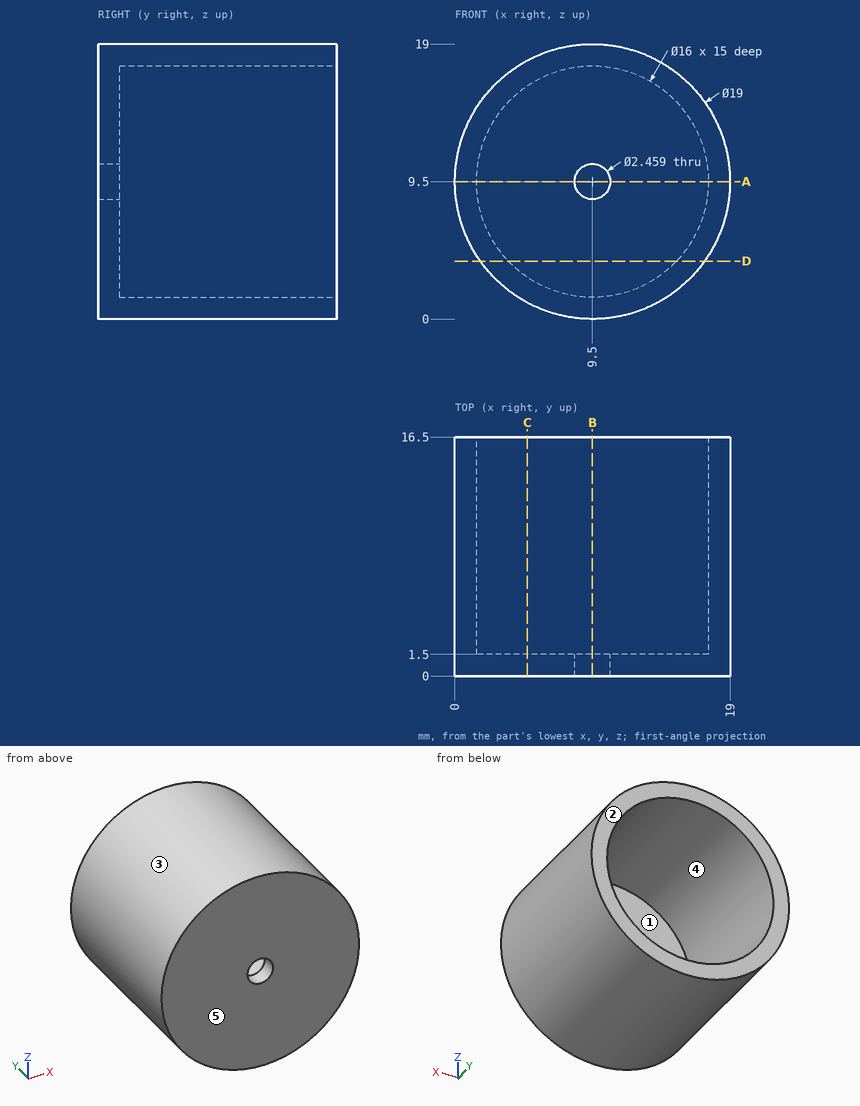
Study the drawing (mm; zero at the part's minimum x, y, z) and answer. A direction names the side the tool comes from. Give positions to 0.01 mm unless a question says otherwise; leave off trailing zeros. Write each loop counter-clockwise with the first axis right and the second up, starting at its lowest first coordinate (ties: lowest second). Pieces come first, ordered by that corner, then holes. Notation, with made-up numbers: M 45.25,88 L 52.25,88 A29 ccw 52.25,115 Z; hole C -5,27 d2. An arc over 180 degrees is marked long. Put each result on its own line as item: value. Start each with the question number.
1. The part is cut by section D-D, the plane z = 4. Give the vertices of the cut face in (x, y), and give its area (3 significant figures).
2. The part is cut by section C-C, the plane x = 5. Give the vertices of the cut face in (y, z), and give its area (3 significant figures).
3. Consider line 1 along Z through (x, y) = (9.5, 0.6); line 2 along Y through (x, z) = (11.5, 12); line 3 along Z through (x, y) = (9.5, 11.25). Determine where each line is inside the solid, lowest interval first.
4. Each of these flat-tipped pins is pushed along its axis until it touches: pin 1 Ø1.5 at (x, y) = (7, 2) entering from -Z; pin 2 Ø1 at (x, y) = (16, 14.5) entering from -Z; pin 3 Ø1.5 at (y, z) = (4, 15) entering from -X. Where does it stop, or does it pass through?
5. Which of the six approach directions +Z, -Z, +X, -X, +Y, -Y give full straight-line access (tool end or side, diameter ignored) to the marked faces 1 and 2?
6. For a pull along X with two mould halves and no side action, classify the marked faces 3, 4 and 5 as released by +X, released by -X, zero draft, split by the parting line, or undercut.
7. The part is cut by section A-A, the plane z = 9.5. Give the vertices of the cut face in (x, y).
8. The part is cut by section B-B, the plane x = 9.5. Give the vertices of the cut face in (y, z), and give its area (3 significant figures).
Final values:
1. outline: M 1.75,0 L 17.25,0 L 17.25,16.5 L 15.31,16.5 L 15.31,1.5 L 3.69,1.5 L 3.69,16.5 L 1.75,16.5 Z
1. area: 81.3 mm²
2. outline: M 0,1.13 L 16.5,1.13 L 16.5,2.89 L 1.5,2.89 L 1.5,16.11 L 16.5,16.11 L 16.5,17.87 L 0,17.87 Z
2. area: 77.7 mm²
3. line 1: z = 0 to 8.27, 10.73 to 19
3. line 2: y = 0 to 1.5
3. line 3: z = 0 to 1.5, 17.5 to 19
4. pin 1: stops at z = 0.16
4. pin 2: stops at z = 2.13
4. pin 3: stops at x = 1.27
5. face 1: +Y
5. face 2: +Z, -Z, +X, -X, +Y
6. face 3: split by the parting line
6. face 4: undercut
6. face 5: zero draft
7. outline: M 0,0 L 8.27,0 L 8.27,1.5 L 1.5,1.5 L 1.5,16.5 L 0,16.5 Z; M 10.73,0 L 19,0 L 19,16.5 L 17.5,16.5 L 17.5,1.5 L 10.73,1.5 Z
8. outline: M 0,0 L 16.5,0 L 16.5,1.5 L 1.5,1.5 L 1.5,8.27 L 0,8.27 Z; M 0,10.73 L 1.5,10.73 L 1.5,17.5 L 16.5,17.5 L 16.5,19 L 0,19 Z
8. area: 69.8 mm²
